from build123d import *

# Parameters (mm, degrees)
SKETCH1_R         = 47.625
EXTRUDE1_DEPTH    = 8.255
SKETCH2_R         = 38.1
EXTRUDE2_DEPTH    = 8.255
SKETCH3_W         = 3.81
SKETCH3_H         = 5.3975
CHAMFER1_SIZE     = 0.635
HOLE1_D           = 2.794
HOLE1_DEPTH       = 8.255
HOLE1_CSINK_D     = 5.334
HOLE1_CSINK_ANGLE = 82
HOLE2_D           = 2.794
HOLE2_DEPTH       = 8.255
HOLE2_CSINK_D     = 5.334
HOLE2_CSINK_ANGLE = 82
HOLE3_D           = 2.794
HOLE3_DEPTH       = 8.255
HOLE3_CSINK_D     = 5.334
HOLE3_CSINK_ANGLE = 82
HOLE4_D           = 2.794
HOLE4_DEPTH       = 8.255
HOLE4_CSINK_D     = 5.334
HOLE4_CSINK_ANGLE = 82
HOLE5_D           = 2.794
HOLE5_DEPTH       = 8.255
HOLE5_CSINK_D     = 5.334
HOLE5_CSINK_ANGLE = 82
HOLE6_D           = 2.794
HOLE6_DEPTH       = 8.255
HOLE6_CSINK_D     = 5.334
HOLE6_CSINK_ANGLE = 82
CHAMFER2_SIZE     = 0.381
CHAMFER3_SIZE     = 0.762


with BuildPart() as part:
    # Sketch1 → Extrude1 (new body)
    with BuildSketch(Plane.XY.offset(12.7)):
        Circle(SKETCH1_R)
    extrude(amount=-EXTRUDE1_DEPTH)

    # Sketch2 → Extrude2 (cut)
    with BuildSketch(Plane.XY.offset(12.7)):
        Circle(SKETCH2_R)
    extrude(amount=-EXTRUDE2_DEPTH, mode=Mode.SUBTRACT)

    # Sketch3 → Cut-Revolve1 (revolve, cut)
    with BuildSketch(Plane.XZ):
        with Locations((45.72, 7.14375)):
            Rectangle(SKETCH3_W, SKETCH3_H)
    revolve(axis=Axis((0, 0, 9.8425), (0, 0, -1)), mode=Mode.SUBTRACT)

    # Chamfer1
    chamfer1_edges = [part.edges().sort_by_distance(p)[0] for p in [
        (-38.1, 0, 12.7),
    ]]
    chamfer(chamfer1_edges, length=CHAMFER1_SIZE)

    # Hole1
    with Locations(Plane.XY.offset(12.7)):
        with Locations((-20.701, -35.855183767)):
            CounterSinkHole(HOLE1_D / 2, HOLE1_CSINK_D / 2, depth=HOLE1_DEPTH, counter_sink_angle=HOLE1_CSINK_ANGLE)

    # Hole2
    with Locations(Plane.XY.offset(12.7)):
        with Locations((-41.402, 0)):
            CounterSinkHole(HOLE2_D / 2, HOLE2_CSINK_D / 2, depth=HOLE2_DEPTH, counter_sink_angle=HOLE2_CSINK_ANGLE)

    # Hole3
    with Locations(Plane.XY.offset(12.7)):
        with Locations((-20.701, 35.855183767)):
            CounterSinkHole(HOLE3_D / 2, HOLE3_CSINK_D / 2, depth=HOLE3_DEPTH, counter_sink_angle=HOLE3_CSINK_ANGLE)

    # Hole4
    with Locations(Plane.XY.offset(12.7)):
        with Locations((20.701, 35.855183767)):
            CounterSinkHole(HOLE4_D / 2, HOLE4_CSINK_D / 2, depth=HOLE4_DEPTH, counter_sink_angle=HOLE4_CSINK_ANGLE)

    # Hole5
    with Locations(Plane.XY.offset(12.7)):
        with Locations((20.701, -35.855183767)):
            CounterSinkHole(HOLE5_D / 2, HOLE5_CSINK_D / 2, depth=HOLE5_DEPTH, counter_sink_angle=HOLE5_CSINK_ANGLE)

    # Hole6
    with Locations(Plane.XY.offset(12.7)):
        with Locations((41.402, 0)):
            CounterSinkHole(HOLE6_D / 2, HOLE6_CSINK_D / 2, depth=HOLE6_DEPTH, counter_sink_angle=HOLE6_CSINK_ANGLE)

    # Chamfer2
    chamfer2_edges = [part.edges().sort_by_distance(p)[0] for p in [
        (-47.625, 0, 9.8425),
    ]]
    chamfer(chamfer2_edges, length=CHAMFER2_SIZE)

    # Chamfer3
    chamfer3_edges = [part.edges().sort_by_distance(p)[0] for p in [
        (-47.625, 0, 12.7),
    ]]
    chamfer(chamfer3_edges, length=CHAMFER3_SIZE)


solid = part.part
Check sheet for the modelled part. Datum: model origin and axes. Units: mm. A direction names the side the tool comes from. Round coordinates to 2 decimals unless told otherwise and drop trailing zeros. Loops run counter-clockwise (first coordinate to the right, second up) from the corner with the lowest first, then second, coordinate; pieces in that order, holes last.
1. Set-up check for faces 4 (the cylindrical face through (20.88, -34.47, 7.79)), 5 (the cylindrical face through (-9.498, 42.773, 7.182)): record each of +Z, -Z, +X, -X, +Y, -Y from which the full face is reachable in a straight line by a thin tool's end or side.
2. Gauge pin test, flat ends, axial feed: pin 1 Ø2 at (y, z) = (24, 5.5) entering from -X; pin 2 Ø1.5 at (x, z) = (31, 6.5) entering from -Y; pin 3 Ø3 at (y, z) = (-35, 11) entering from -X. Record the tip position at first contact, or that the pin passes through.
3. Sectioned sample at A-A on x = 0. Record the boundary of the cut face in (y, z) (1 decimal).
4. Sectioned sample at B-B on z = 7.75. Record the boundary of the cut face in (x, y) (3 decimals).
5. Scan lines: probe 1 along X at (y, z) = (-35, 7.75); probe 2 along Y at (x, z) = (20, 11.5); probe 3 along Y at (x, z) = (0, 8.75) (3 decimals). Record each from-to range of solid material in increasing order.
6. Mould release check, pull along X, two halves, no side actions. Record for faces 1 (the cylindrical face through (-37.794, -28.979, 11.093)), 2 (the cylindrical face through (-22.033, 36.275, 7.794)), 3 (the flat face through (-14, 42, 9.842)): released by +X, released by -X, zero draft, split by the parting line, or undercut.
Recorded:
1. face 4: +Z, -Z
1. face 5: -Z
2. pin 1: stops at x = -37.29
2. pin 2: stops at y = -31.7
2. pin 3: stops at x = -33.85
3. outline: (-47.6, 10.2) - (-47.2, 9.8) - (-43.8, 9.8) - (-43.8, 4.4) - (-38.1, 4.4) - (-38.1, 12.1) - (-38.7, 12.7) - (-46.9, 12.7) - (-47.6, 11.9) - close; (38.1, 4.4) - (43.8, 4.4) - (43.8, 9.8) - (47.2, 9.8) - (47.6, 10.2) - (47.6, 11.9) - (46.9, 12.7) - (38.7, 12.7) - (38.1, 12.1) - close
4. outline: circle Ø87.63 at (0, 0); hole circle Ø2.794 at (-41.402, 0); hole circle Ø76.2 at (0, 0); hole circle Ø2.794 at (-20.701, -35.855); hole circle Ø2.794 at (-20.701, 35.855); hole circle Ø2.794 at (20.701, -35.855); hole circle Ø2.794 at (20.701, 35.855); hole circle Ø2.794 at (41.402, 0)
5. probe 1: x = -26.36 to -21.81, -19.6 to -15.05, 15.05 to 19.6, 21.81 to 26.36
5. probe 2: y = -43.22 to -37.32, -34.39 to -32.43, 32.43 to 34.39, 37.32 to 43.22
5. probe 3: y = -43.815 to -38.1, 38.1 to 43.815
6. face 1: split by the parting line
6. face 2: undercut
6. face 3: zero draft
